CAD build for the part. Positions are in the model's coordinates, mm. Face numbers are marked on the shaded views. A direction names the side the tool comes from. Round coordinates to 2 decimals unless told otherwise and drop trailing zeros. Order: outer loops, then holes, each group sorted by start corner. A loop starts at its lowest first (then second) coordinate and runs counter-clockwise, first axis right, second up. Notation, with made-up numbers: (-17, 39.5) -> (25, 39.5) arc R7 ccw to (25, 52.5) -> close; hole circle Ø4 at (27.5, -13). An arc over 180 degrees is marked (long way). Return JSON: item names as keys, results as strings. Group by question number.
Q1. Mould opens along X. For the marked faces 3, 4 and 5 say: +X half, -X half, draft (parallel to the pull), parting line (faces both ways), or undercut.
Q2. Cut at B-B (x = -836). Write the cut outline in (y, z), then the cut area to 3 significant figures.
Q3. Which spindle directions (+Z, -Z, +X, -X, +Y, -Y) get a long thin tool onto all of the face, cutting with end or side? Do the marked faces 1 and 2. Say none if no direction does.
Q4. Flat gauge pins, fed straight in: pin 1 (17.5 mm diameter, centred on x = -193.5, y = -1035, fed in from +Z); pin 2 (1.5 mm diameter, centred on x = 283.5, z = 381.5, fed in from -Y); pin 3 (10 mm diameter, centred on x = -457.5, y = -702.5, fed in from +Z). Where does each tip first touch, or does it go through?
Q5. Cut at A-A (z = 246.5). Write the cut outline in (x, y).
Q6. Cut at C-C (z = 8.5). Write the cut outline in (x, y).
Q7. Cut at D-D (y = -843). Write the cut outline in (x, z), then the cut area to 3 significant figures.
Q8. Probe line 1 along X through (y, z) = (-222.5, -40.5); line 2 along Y through (x, z) = (424, 424); line 3 along Y through (x, z) = (27, 72.5). List the from-to ranges inside material, lowest first.
from build123d import *

# Parameters (mm, degrees)
F0_W     = 1950
F0_H     = 35
F1_DEPTH = 1050
F0_H_2   = 135
F0_H_3   = 165
F2_DEPTH = 35
F3_W     = 35
F3_H     = 35
F4_DEPTH = 975


with BuildPart() as f1:
    # F0 (on Front) → F1 (new body)
    with BuildSketch(Plane.XZ):
        Polygon((-975, -65), (-975, 100), (-975, 365), (-975, 500), (-1010, 500), (-1010, -100), (-975, -100), align=None)
        with Locations((0, -82.5)):
            Rectangle(F0_W, F0_H)
        Polygon((975, 365), (975, 100), (975, -65), (975, -100), (1010, -100), (1010, 500), (975, 500), align=None)
    extrude(amount=F1_DEPTH)

    # F0 (on Front) → F2 (join)
    with BuildSketch(Plane.XZ):
        Polygon((-975, -65), (-975, 100), (-975, 365), (-975, 500), (-1010, 500), (-1010, -100), (-975, -100), align=None)
        Polygon((975, 365), (975, 100), (975, -65), (975, -100), (1010, -100), (1010, 500), (975, 500), align=None)
        with Locations((0, -82.5)):
            Rectangle(F0_W, F0_H)
        with Locations((0, 432.5)):
            Rectangle(F0_W, F0_H_2)
        with Locations((0, 17.5)):
            Rectangle(F0_W, F0_H_3)
    extrude(amount=F2_DEPTH)

    # F3 (on Right) → F4 (join, symmetric)
    with BuildSketch(Plane.YZ):
        Polygon((-1015, 100), (-1050, 100), (-1050, -100), (-1015, -100), (-1015, -65), align=None)
        with Locations((-997.5, -82.5)):
            Rectangle(F3_W, F3_H)
        with Locations((-52.5, -82.198536)):
            Rectangle(F3_W, F3_H)
    extrude(amount=F4_DEPTH, both=True)


solid = f1.part
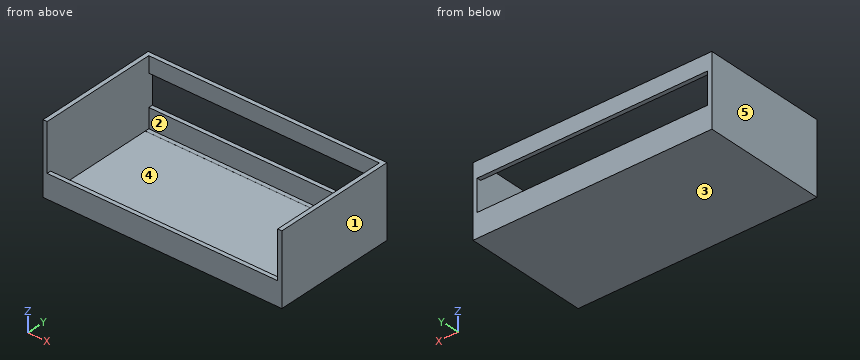
Solution:
{
 "1": {"face 3": "draft", "face 4": "undercut", "face 5": "-X half"},
 "2": {"outline": "(-1050, -100) -> (0, -100) -> (0, 100) -> (-35, 100) -> (-35, -64.7) -> (-70, -64.7) -> (-70, -65) -> (-1015, -65) -> (-1015, 100) -> (-1050, 100) -> close; (-35, 365) -> (0, 365) -> (0, 500) -> (-35, 500) -> close", "area": "53,000 mm²"},
 "3": {"face 1": "+Z, -Z, +X, +Y, -Y", "face 2": "+Z"},
 "4": {"pin 1": "stops at z = 100", "pin 2": "stops at y = -35", "pin 3": "stops at z = -65"},
 "5": {"outline": "(-1010, -1050) -> (-975, -1050) -> (-975, 0) -> (-1010, 0) -> close; (975, -1050) -> (1010, -1050) -> (1010, 0) -> (975, 0) -> close"},
 "6": {"outline": "(-1010, -1050) -> (1010, -1050) -> (1010, 0) -> (-1010, 0) -> close; hole (-975, -1015) -> (975, -1015) -> (975, -35) -> (-975, -35) -> close"},
 "7": {"outline": "(-1010, -100) -> (1010, -100) -> (1010, 500) -> (975, 500) -> (975, -65) -> (-975, -65) -> (-975, 500) -> (-1010, 500) -> close", "area": "110,000 mm²"},
 "8": {"line 1": "x = -1010 to -975, 975 to 1010", "line 2": "y = -35 to 0", "line 3": "y = -1050 to -1015, -35 to 0"}
}
